Autodesk Inventor part; units mm, degrees
ref_plane "YZ Plane" through (0, 0, 0) normal (1, 0, 0) x (0, 1, 0)
ref_plane "XZ Plane" through (0, 0, 0) normal (0, 1, 0) x (-1, 0, 0)
ref_plane "XY Plane" through (0, 0, 0) normal (0, 0, 1) x (1, 0, 0)
sketch "Esquisse1" plane through (0, 0, 0) normal (0, 1, 0) x (-1, 0, 0)
  line L0 (0, 0) -> (0, -30)
  line L1 (0, -30) -> (10.6495, -30)
  line L2 (0, -30) -> (10.6495, -30) construction
  line L3 (0, -30) -> (-10.6495, -30)
  line L4 (0, 0) -> (5, 0)
  line L5 (0, 0) -> (-5, 0)
  line L6 (-5, 0) -> (-10.6495, -30)
  line L7 (5, 0) -> (10.6495, -30)
  line L8 (5, 0) -> (8, 0)
  line L9 (10.6495, -30) -> (13.6495, -30)
  line L10 (13.6495, -30) -> (8, 0)
  line L11 (-10.6495, -30) -> (-13.6495, -30)
  line L12 (-5, 0) -> (-8, 0)
  line L13 (-8, 0) -> (-13.6495, -30)
  line L14 (0, 0) -> (0, 2)
  line L15 (0, 2) -> (8, 2)
  line L16 (8, 2) -> (8, 0)
  line L17 (0, 2) -> (-8, 2)
  line L18 (-8, 2) -> (-8, 0)
  dimension "d0" = 30
  dimension "d1" = 10.6495
  dimension "d2" = 0
  dimension "d3" = 10.6495
  dimension "d4" = 5
  dimension "d5" = 5
  dimension "d7" = 3
  dimension "d8" = 3
  dimension "d9" = 3
  dimension "d10" = 3
  dimension "d11" = 2
extrude "Extrusion1" add sketch "Esquisse1" along normal blind 12 contours L14 L15 L16 L8 L4 | L5 L12 L18 L17 L14 | L8 L10 L9 L7 | L6 L11 L13 L12
sketch "Esquisse2" plane through (0, 0, 0) normal (0, -1, 0) x (1, 0, 0)
  line L0 (-5, 0) -> (-10.6495, -30)
  line L1 (-5, 0) -> (-10.6495, -30)
  line L2 (10.6495, -30) -> (5, 0)
  line L3 (-10.6495, -30) -> (10.6495, -30)
  line L4 (10.6495, -30) -> (5, 0)
  line L5 (5, 0) -> (-5, 0)
  point P0 (0, 0)
extrude "Extrusion2" add sketch "Esquisse2" against normal blind 0.99
sketch "Esquisse3" plane through (0, 12, 0) normal (0, 1, 0) x (1, 0, 0)
  line L0 (5, 0) -> (-5, 0)
  line L1 (5, 0) -> (-5, 0)
  line L2 (-10.6495, 30) -> (-13.6495, 30)
  line L3 (-5, 0) -> (-10.6495, 30)
  line L4 (10.6495, 30) -> (5, 0)
  line L5 (-10.6495, 30) -> (10.6495, 30)
  line L6 (10.6495, 30) -> (5, 0)
  point P0 (0, 0)
extrude "Extrusion3" add sketch "Esquisse3" against normal blind 0.99
sketch "Esquisse4" plane through (0, 12, 0) normal (0, 1, 0) x (1, 0, 0)
  line L0 (0, 0) -> (0, 30)
  line L1 (13.6495, 30) -> (-13.6495, 30)
  line L2 (0, 0) -> (0, 10)
  line L3 (0, 10) -> (0, 20)
  dimension "d18" = 10
  dimension "d19" = 10
hole "Perçage1" at (0, 12, -10) at (0, 12, -20) direction (0, -1, 0) diameter 4.134 end through all
sketch "Esquisse5" plane through (0, 12, 0) normal (0, 1, 0) x (1, 0, 0)
  line L0 (-8, -2) -> (8, -2)
  line L1 (-8, -2) -> (-8, -7)
  line L2 (-8, -7) -> (8, -7)
  line L3 (8, -7) -> (8, -2)
  arc A0 (-8, -7) -> (8, -7) centre (0, -7) ccw
  point P0 (0, 0)
  dimension "d27" = 5
extrude "Extrusion4" add sketch "Esquisse5" against normal blind 1
fillet "Congé1" radius 2.5 1 edges at (0, 11, 2)
sketch "Esquisse7" plane through (0, 12, 0) normal (0, 1, 0) x (1, 0, 0)
  line L0 (0, 0) -> (0, -10)
  dimension "d31" = 10
sketch "Esquisse8" plane through (0, 0, 0) normal (0, -1, 0) x (1, 0, 0)
  line L0 (-8, 2) -> (8, 2)
  line L1 (-8, 7) -> (-8, 2)
  line L2 (8, 7) -> (8, 0)
  line L3 (8, 2) -> (8, 7)
  line L4 (-8, 2) -> (8, 2)
  arc A0 (8, 7) -> (-8, 7) centre (0, 7) ccw
  point P0 (0, 0)
extrude "Extrusion5" add sketch "Esquisse8" against normal blind 1
fillet "Congé2" radius 2.5 1 edges at (0, 1, 2)
hole "Perçage2" at (0, 12, 10) direction (0, -1, 0) diameter 4.134 end through all
properties part number "Fixation_rotule_axe_centrale"
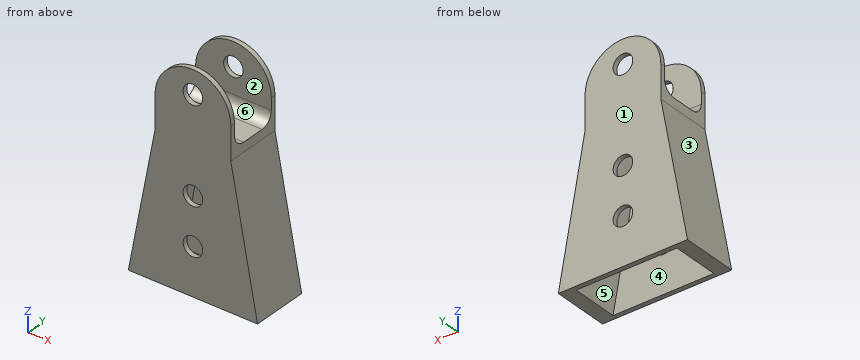
Check sheet for the modelled part. Datum: model origin and axes. Units: mm. Face numbers are marked on the shaded views. A direction names the side the tool comes from. Round coordinates to 2 decimals unless told otherwise and drop trailing zeros. Order: outer loops, then holes, each group sorted by start corner. A loop starts at its lowest first (then second) coordinate and runs counter-clockwise, first axis right, second up.
(1) Cross-section at A-A, the plane z = 3. Enter the section's corners in (x, y).
(2) Cross-section at C-C, the plane x = 0. State how many separate pieces and enclosed holes the cut face has, and give its area (3 significant figures).
(3) Cross-section at B-B, the plane y = 7.25. Enter the section's corners in (x, z).
(4) Go/stop test with flat-tipped pins: P1, Ø1, axis at x = -3, y = 9.5, coming from the -Z side; P2, Ø4, axis at y = 6.5, z = -6, coming from the +X side; P3, Ø4, axis at x = 4, y = 5.5, coming from the +Z side. Record where each tip stops, or that it passes through.
(5) Draft check along X on the marked faces 3, 4, 5 and 6. Enter one of: pulls with the +X half, pulls with the -X half, needs draft (parallel to the pull), parting line crosses it, or undercut.
(6) Access from +Z, -Z, +X, -X, +Y, -Y to the whole of each face (thin tool, end or side, straight path). Record for the marked faces 1 and 2.
(7) Scan lines: probe 1 along Z at (x, y) = (0, 11.4); probe 2 along Y at (x, z) = (1, -25); probe 3 along X at (y, z) = (5.25, -13.5). Record each from-to range of solid material in increasing order.
(8) Cross-section at D-D, the plane z = 10. Enter the section's corners in (x, y), and give its area (3 significant figures).
Check sheet entries:
1. outline: (-8, 0) - (8, 0) - (8, 1.5) - (-8, 1.5) - close; (-8, 10.5) - (8, 10.5) - (8, 12) - (-8, 12) - close
2. separate pieces: 7
2. enclosed holes: 0
2. area: 87.4 mm2
3. outline: (-13.65, -30) - (-10.65, -30) - (-5, 0) - (5, 0) - (10.65, -30) - (13.65, -30) - (8, 0) - (8, 2) - (-8, 2) - (-8, 0) - close
4. P1: stops at z = 0
4. P2: stops at x = 9.51
4. P3: stops at z = 2
5. face 3: pulls with the -X half
5. face 4: undercut
5. face 5: undercut
5. face 6: needs draft
6. face 1: +Z, -Z, +X, -X, +Y
6. face 2: +Z, +X, -X
7. probe 1: z = -30 to -22.07, -17.93 to -12.07, -7.93 to 7.93, 12.07 to 15
7. probe 2: y = 0 to 0.99, 11.01 to 12
7. probe 3: x = -10.54 to -7.54, 7.54 to 10.54
8. outline: (-7.42, 0) - (-2.07, 0) - (-2.07, 1) - (-7.42, 1) - close; (-7.42, 11) - (-2.07, 11) - (-2.07, 12) - (-7.42, 12) - close; (2.07, 0) - (7.42, 0) - (7.42, 1) - (2.07, 1) - close; (2.07, 11) - (7.42, 11) - (7.42, 12) - (2.07, 12) - close
8. area: 21.4 mm2
